Work out the finished part from the listing and answer in its coordinate system (mm). A direction names the side the tool comes from. Give positions to 0.01 mm unless a question says otherwise; leave off trailing zeros. Write each loop counter-clockwise with the first axis right and the second up, starting at its lowest first coordinate (ties: lowest second). Pieces come first, ordered by that corner, then holes. Notation, with made-up numbers: (3, -28.5) - (40, -28.5) arc R34 ccw to (40, 2.5) - close; hole circle Ø5 at (74, 31). An arc over 180 degrees is marked (long way). Write item = value, one per line.
from build123d import *

# Parameters (mm, degrees)
SKETCH1_R            = 8.5
BOSS_EXTRUDE1_DEPTH  = 6
BOSS_EXTRUDE2_DEPTH  = 1.25
SKETCH3_R            = 1.6
SKETCH3_R_2          = 0.85
BOSS_EXTRUDE3_DEPTH  = 0.5
CUT_EXTRUDE1_START   = -1.25
SKETCH5_R            = 0.85
CUT_EXTRUDE1_DEPTH   = 1.25
BOSS_EXTRUDE5_START  = -0.5
BOSS_EXTRUDE5_DEPTH  = 0.5
BOSS_EXTRUDE6_START  = 0.5
SKETCH8_R            = 1.6
SKETCH8_R_2          = 0.85
BOSS_EXTRUDE6_DEPTH  = 0.5
FILLET2_R            = 0.5
BOSS_EXTRUDE7_DEPTH  = 0.1
BOSS_EXTRUDE8_DEPTH  = 1
SKETCH11_R           = 3.5
BOSS_EXTRUDE9_DEPTH  = 7
SKETCH12_R           = 3
BOSS_EXTRUDE10_DEPTH = 3
SKETCH14_R           = 3
BOSS_EXTRUDE11_DEPTH = 6
CUT_EXTRUDE2_DEPTH   = 7
BOSS_EXTRUDE12_DEPTH = 0.5
BOSS_EXTRUDE13_DEPTH = 2.5
FILLET4_R            = 1


# Read off the part's stored shape, not the designer's step: Boss-Extrude13
with BuildPart() as part:
    # Sketch1 → Boss-Extrude1 (new body)
    with BuildSketch(Plane.XY):
        Circle(SKETCH1_R)
    extrude(amount=-BOSS_EXTRUDE1_DEPTH)

    # Sketch2 → Boss-Extrude2 (add)
    with BuildSketch(Plane.XY):
        with BuildLine():
            Line((8.75, 0), (8.75, -11.25))
            Line((8.75, -11.25), (-8.75, -11.25))
            Line((-8.75, -11.25), (-8.75, 0))
            ThreePointArc((-8.75, 0), (0, 8.75), (8.75, 0))
        make_face()
    extrude(amount=BOSS_EXTRUDE2_DEPTH)

    # Sketch3 → Boss-Extrude3 (add)
    # profile 1 of 3: a face of its own
    with BuildSketch(Plane.XY.offset(1.25)):
        with Locations((0, -8.75)):
            Circle(SKETCH3_R)
        with Locations((0, -8.75)):
            Circle(SKETCH3_R_2, mode=Mode.SUBTRACT)
    # profile 2 of 3: a face of its own
    with BuildSketch(Plane.XY.offset(1.25)):
        with Locations((6.25, -8.75)):
            Circle(SKETCH3_R)
        with Locations((6.25, -8.75)):
            Circle(SKETCH3_R_2, mode=Mode.SUBTRACT)
    # profile 3 of 3: a face of its own
    with BuildSketch(Plane.XY.offset(1.25)):
        with Locations((-6.25, -8.75)):
            Circle(SKETCH3_R)
        with Locations((-6.25, -8.75)):
            Circle(SKETCH3_R_2, mode=Mode.SUBTRACT)
    extrude(amount=BOSS_EXTRUDE3_DEPTH)

    # Sketch5 → Cut-Extrude1 (cut)
    with BuildSketch(Plane.XY.offset(1.25).offset(CUT_EXTRUDE1_START)):
        with Locations((-6.25, -8.75)):
            Circle(SKETCH5_R)
        with Locations(Location((0, -8.75, 0), (0, 0, 160.215255231))):
            Circle(SKETCH5_R)
        with Locations((6.25, -8.75)):
            Circle(SKETCH5_R)
    extrude(amount=CUT_EXTRUDE1_DEPTH, mode=Mode.SUBTRACT)

    # Sketch6 → Boss-Extrude5 (add)
    with BuildSketch(Plane.XY.offset(BOSS_EXTRUDE5_START)):
        with BuildLine():
            Line((-6.75, -15.85), (-6.75, -10.269868415))
            ThreePointArc((-6.75, -10.269868415), (-6.25, -10.35), (-5.75, -10.269868415))
            Line((-5.75, -10.269868415), (-5.75, -15.85))
            ThreePointArc((-5.75, -15.85), (-6.25, -16.35), (-6.75, -15.85))
        make_face()
        with BuildLine():
            Line((-0.5, -15.85), (-0.5, -10.269868415))
            ThreePointArc((-0.5, -10.269868415), (0, -10.35), (0.5, -10.269868415))
            Line((0.5, -10.269868415), (0.5, -15.85))
            ThreePointArc((0.5, -15.85), (0, -16.35), (-0.5, -15.85))
        make_face()
        with BuildLine():
            Line((5.75, -15.85), (5.75, -10.269868415))
            ThreePointArc((5.75, -10.269868415), (6.25, -10.35), (6.75, -10.269868415))
            Line((6.75, -10.269868415), (6.75, -15.85))
            ThreePointArc((6.75, -15.85), (6.25, -16.35), (5.75, -15.85))
        make_face()
    extrude(amount=BOSS_EXTRUDE5_DEPTH)

    # Sketch8 → Boss-Extrude6 (add)
    # profile 1 of 3: a face of its own
    with BuildSketch(Plane(origin=(0, 0, 0), x_dir=(-1, 0, 0), z_dir=(0, 0, -1)).offset(BOSS_EXTRUDE6_START)):
        with Locations(Location((-6.25, -8.75, 0), (0, 0, 180))):
            Circle(SKETCH8_R)
        with Locations(Location((-6.25, -8.75, 0), (0, 0, 180))):
            Circle(SKETCH8_R_2, mode=Mode.SUBTRACT)
    # profile 2 of 3: a face of its own
    with BuildSketch(Plane(origin=(0, 0, 0), x_dir=(-1, 0, 0), z_dir=(0, 0, -1)).offset(BOSS_EXTRUDE6_START)):
        with Locations(Location((0, -8.75, 0), (0, 0, 180))):
            Circle(SKETCH8_R)
        with Locations(Location((0, -8.75, 0), (0, 0, 19.784744769))):
            Circle(SKETCH8_R_2, mode=Mode.SUBTRACT)
    # profile 3 of 3: a face of its own
    with BuildSketch(Plane(origin=(0, 0, 0), x_dir=(-1, 0, 0), z_dir=(0, 0, -1)).offset(BOSS_EXTRUDE6_START)):
        with Locations(Location((6.25, -8.75, 0), (0, 0, 180))):
            Circle(SKETCH8_R)
        with Locations(Location((6.25, -8.75, 0), (0, 0, 180))):
            Circle(SKETCH8_R_2, mode=Mode.SUBTRACT)
    extrude(amount=-BOSS_EXTRUDE6_DEPTH)

    # Fillet2
    fillet2_edges = [part.edges().sort_by_distance(p)[0] for p in [
        (-1.6, -8.75, 1.75),
        (4.65, -8.75, 1.75),
        (-7.85, -8.75, 1.75),
    ]]
    fillet(fillet2_edges, radius=FILLET2_R - 0.0001)  # a hair under: the kernel refuses the full size

    # Sketch9 → Boss-Extrude7 (add)
    with BuildSketch(Plane.XY.offset(1.25)):
        with BuildLine():
            Line((-7.180703308, 5), (7.180703308, 5))
            ThreePointArc((7.180703308, 5), (8.75, 0), (7.180703308, -5))
            Line((7.180703308, -5), (-7.180703308, -5))
            ThreePointArc((-7.180703308, -5), (-8.75, 0), (-7.180703308, 5))
        make_face()
    extrude(amount=BOSS_EXTRUDE7_DEPTH)

    # Sketch10 → Boss-Extrude8 (add)
    with BuildSketch(Plane.XY.offset(1.35)):
        with BuildLine():
            Line((2.291287847, 5), (-2.291287847, 5))
            ThreePointArc((-2.291287847, 5), (-5.5, 0), (-2.291287847, -5))
            Line((-2.291287847, -5), (2.291287847, -5))
            ThreePointArc((2.291287847, -5), (5.5, 0), (2.291287847, 5))
        make_face()
    extrude(amount=BOSS_EXTRUDE8_DEPTH)

    # Sketch11 → Boss-Extrude9 (add)
    with BuildSketch(Plane.XY.offset(2.35)):
        Circle(SKETCH11_R)
    extrude(amount=BOSS_EXTRUDE9_DEPTH)

    # Sketch12 → Boss-Extrude10 (add)
    with BuildSketch(Plane.XY.offset(9.35)):
        Circle(SKETCH12_R)
    extrude(amount=BOSS_EXTRUDE10_DEPTH)

    # Sketch13 → Cut-Revolve2 (revolve, cut)
    with BuildSketch(Plane(origin=(0, 0, 0), x_dir=(1, 0, 0), z_dir=(0, 1, 0))):
        Polygon((2.076228104, -11.010865145), (2.076228104, -12.35), (3, -12.35), (3, -10.050978955), align=None)
    revolve(axis=Axis((0, 0, 12.35), (0, 0, -1)), mode=Mode.SUBTRACT)

    # Sketch14 → Boss-Extrude11 (add)
    with BuildSketch(Plane.XY.offset(12.35)):
        Circle(SKETCH14_R)
    extrude(amount=BOSS_EXTRUDE11_DEPTH)

    # Sketch15 → Cut-Extrude2 (cut)
    with BuildSketch(Plane.XY.offset(18.35)):
        Polygon((-3.122971825, 2.701860488), (2.385287248, -3.377006001), (3.122971825, -2.701860488), (-2.385287248, 3.377006001), align=None)
    extrude(amount=-CUT_EXTRUDE2_DEPTH, mode=Mode.SUBTRACT)

    # Sketch16 → Boss-Extrude12 (add)
    with BuildSketch(Plane.XY.offset(1.35)):
        with BuildLine():
            Line((-8.442304188, 2.3), (-5.333008063, 1.345))
            ThreePointArc((-5.333008063, 1.345), (-5.5, 0), (-5.333008063, -1.345))
            Line((-5.333008063, -1.345), (-8.442304188, -2.3))
            ThreePointArc((-8.442304188, -2.3), (-8.749950498, 0), (-8.442304188, 2.3))
        make_face()
    extrude(amount=BOSS_EXTRUDE12_DEPTH)

    # Boss-Extrude13 outline → Boss-Extrude13 (add)
    with BuildSketch(Plane.XY.offset(1.85)):
        with BuildLine():
            ThreePointArc((-8.701900167, 0.915807021), (-8.749950498, 0), (-8.701900167, -0.915807021))
            ThreePointArc((-8.701900167, -0.915807021), (-8.085984441, -1.372236974), (-7.571237459, -0.804155968))
            Line((-7.571237459, -0.804155968), (-7.571237459, 0.804155968))
            ThreePointArc((-7.571237459, 0.804155968), (-8.085984441, 1.372236974), (-8.701900167, 0.915807021))
        make_face()
    extrude(amount=BOSS_EXTRUDE13_DEPTH)

    # Fillet4
    fillet4_edges = [part.edges().sort_by_distance(p)[0] for p in [
        (-8.5, 0, -6),
    ]]
    fillet(fillet4_edges, radius=FILLET4_R)


solid = part.part
1. Given pin 1 (1.6 mm diameter, centred on x = 0, y = -13.5, fed in from -Z); pin 2 (0.6 mm diameter, centred on x = -8, y = 0, fed in from +Z); pin 3 (2 mm diameter, centred on x = 2.5, z = 1, fed in from +Y), each flat-ended and moving along its own axis, determine where each tip first touches the part or whether it passes through.
Solution:
pin_1 = -0.5
pin_2 = 4.35
pin_3 = 8.62
2. A tool of negligible diameter and unlimited length cuts with its end or side. For faces 1 (the cylindrical face through (-8.098, -1.373, 3.082)), 2 (the cylindrical face through (4.57, 7.167, -2.465)), 3 (the flat face through (-6.91, 1.83, 1.6)), 4 (the flat face through (3, 1, 9.35)), from which of +Z, -Z, +X, -X, +Y, -Y can it reach the whole face along a straight path? Write none if from no direction.
Solution:
face_1 = +Z, -Y
face_2 = -Z
face_3 = +Z, +Y
face_4 = +Z
3. Find section A-A, the plane z = 16.5. Give the vertices of the cut face in (x, y).
Solution:
outline = (-2.36, 1.86) arc R3 ccw to (1.62, -2.53) - close; (-1.62, 2.53) - (2.36, -1.86) arc R3 ccw to start
4. Find section B-B, the plane z = 6.5. Give the vertices of the cut face in (x, y), then the cut area to 3 significant figures.
Solution:
outline = circle Ø7 at (0, 0)
area = 38.5 mm^2
5. For a pull along Y with two mould halves and no side action, classify faces 5 (the flat face through (0, -7, 1.25)), 6 (the cylindrical face through (-2.26, -1.97, 15.31)), 7 (the flat face through (6, -14, 0)), 8 (the cylindrical face through (6.19, -7.15, -0.25)) as pulls with the +Y half, pulls with the -Y half, needs draft (parallel to the pull), parting line crosses it, or undercut.
Solution:
face_5 = undercut
face_6 = parting line crosses it
face_7 = needs draft
face_8 = undercut
6. Straight lines are drawn through the part: line 1 (X direction, y = -8.75, z = -0.15); line 2 (Y direction, x = 0, z = 0.65); line 3 (Y direction, x = -6.25, z = 1.2). For each, find the intervals that lie inside material, in ascending order.
Solution:
line_1 = -7.85 to -7.1, -5.4 to -4.65, -1.6 to -0.85, 0.85 to 1.6, 4.65 to 5.4, 7.1 to 7.85
line_2 = -11.25 to -9.6, -7.9 to 8.75
line_3 = -11.25 to -9.6, -7.9 to 6.12
7. Find section C-C, the plane z = -3.75. Give the vertices of the cut face in (x, y), then the cut area to 3 significant figures.
Solution:
outline = circle Ø17 at (0, 0)
area = 227 mm^2
